from build123d import *

# Parameters (mm, degrees)
RESSALTO_EXTRUS_O1_DEPTH = 55
ESBO_O3_W                = 15
ESBO_O3_H                = 5
ESBO_O3_R                = 1.65
RESSALTO_EXTRUS_O2_DEPTH = 10


with BuildPart() as part:
    # Esboço1 → Ressalto-extrusão1 (new body)
    with BuildSketch(Plane.XY):
        with BuildLine():
            Line((0, 35), (0, -35))
            Line((0, -35), (13.5, -35))
            ThreePointArc((13.5, -35), (15.581665999, -34.780933834), (17.572127481, -34.133333333))
            Line((17.572127481, -34.133333333), (16.554095611, -31.85))
            ThreePointArc((16.554095611, -31.85), (6, -25), (16.554095611, -18.15))
            Line((16.554095611, -18.15), (17.572127481, -15.866666667))
            ThreePointArc((17.572127481, -15.866666667), (15.581665999, -15.219066166), (13.5, -15))
            Line((13.5, -15), (6, -15))
            Line((6, -15), (6, 15))
            Line((6, 15), (13.5, 15))
            ThreePointArc((13.5, 15), (15.581665999, 15.219066166), (17.572127481, 15.866666667))
            Line((17.572127481, 15.866666667), (16.554095611, 18.15))
            ThreePointArc((16.554095611, 18.15), (6, 25), (16.554095611, 31.85))
            Line((16.554095611, 31.85), (17.572127481, 34.133333333))
            ThreePointArc((17.572127481, 34.133333333), (15.581665999, 34.780933834), (13.5, 35))
            Line((13.5, 35), (0, 35))
        make_face()
    extrude(amount=RESSALTO_EXTRUS_O1_DEPTH)

    # Esboço3 → Ressalto-extrusão2 (add)
    with BuildSketch(Plane(origin=(6, 0, 0), x_dir=(0, 0, -1), z_dir=(1, 0, 0))):
        with Locations((-43.5, 15)):
            Rectangle(ESBO_O3_W, ESBO_O3_H)
        with Locations((-47.5, 15)):
            Circle(ESBO_O3_R, mode=Mode.SUBTRACT)
        with Locations((-39.5, 15)):
            Circle(ESBO_O3_R, mode=Mode.SUBTRACT)
    extrude(amount=RESSALTO_EXTRUS_O2_DEPTH)


solid = part.part
The model under review builds one solid part; all positions refer to its coordinate system, in mm. A direction names the side the tool comes from. Give positions to 0.01 mm unless a question says otherwise; leave off trailing zeros. Write each loop counter-clockwise with the first axis right and the second up, starting at its lowest first coordinate (ties: lowest second). Pieces come first, ordered by that corner, then holes.
1. Add section A-A, the plane x = 12.75. Write out the cut boundary in (y, z), plus the area to 3 significant figures.
2. Wall thickness on L1, parallel to Y at x = 13.5, z = 34; L2, parallel to Y at x = 8.25, z = 49.5; L3, parallel to Y at x = 9.25, z = 47.5: over which ranges is each line inside the solid? List them lowest first.
3. For P1, Ø10, axis at y = -4, z = 33.5, coming from the +X side; P2, Ø5, axis at x = 9, y = 1.5, coming from the +Z side; P3, Ø0.8, axis at x = 12, y = 13.5, coming from the +Z side; P4, Ø1.4, axis at x = 8.5, y = 13.5, coming from the -Z side, all flat-tipped, find the tip position at first contact; note any pin that passes through.
4. Tool access review of faces 4 (the flat face through (10, 15, 18)), 5 (the flat face through (17.06, 32.98, 27.12)), 6 (the cylindrical face through (15.553, 15.213, 27.115)): name each direction out of +Z, -Z, +X, -X, +Y, -Y from which nothing blocks a thin tool from reaching the whole face with its end or side.
5. Add section B-B, the plane z = 39.5. Write out the cut boundary in (x, y).
6. Add section C-C, the plane x = 7.75. Write out the cut boundary in (y, z), plus the area to 3 significant figures.
7. Add section D-D, the plane y = 25. Write out the cut boundary in (x, z).
8. Draft analysis for pull direction Z (two halves, no side actions). For faces 1 (the flat face through (6, 14, 39)), 2 (the flat face through (17.07, 16.99, 27.12)), 3 (the flat face through (11, 14, 36)), state which applies: +Z half, -Z half, draft (parallel to the pull), parting line (faces both ways), or undercut.
Worked answers:
1. outline: (-35, 0) - (-32.46, 0) - (-32.46, 55) - (-35, 55) - close; (-17.54, 0) - (-15, 0) - (-15, 55) - (-17.54, 55) - close; (12.5, 36) - (15, 36) - (15, 0) - (17.54, 0) - (17.54, 55) - (15, 55) - (15, 51) - (12.5, 51) - close; (32.46, 0) - (35, 0) - (35, 55) - (32.46, 55) - close; hole (15, 37.85) - (15, 41.15) arc R1.65 ccw to start; hole (15, 45.85) - (15, 49.15) arc R1.65 ccw to start
1. area: 587 mm2
2. L1: y = -35 to -32.5, -17.5 to -15, 15 to 17.5, 32.5 to 35
2. L2: y = -35 to -30.36, -19.64 to -15, 12.5 to 19.64, 30.36 to 35
2. L3: y = -35 to -31.18, -18.82 to -15, 12.5 to 13.35, 15 to 18.82, 31.18 to 35
3. P1: stops at x = 6
3. P2: passes through
3. P3: stops at z = 51
3. P4: stops at z = 36
4. face 4: -Z, +X
4. face 5: +Z, -Z, +X
4. face 6: +X
5. outline: (0, -35) - (13.5, -35) arc R10 ccw to (17.57, -34.13) - (16.55, -31.85) arc R7.5 cw (long way) to (16.55, -18.15) - (17.57, -15.87) arc R10 ccw to (13.5, -15) - (6, -15) - (6, 12.5) - (16, 12.5) - (16, 13.35) - (6, 13.35) - (6, 15) - (13.5, 15) arc R10 ccw to (17.57, 15.87) - (16.55, 18.15) arc R7.5 cw (long way) to (16.55, 31.85) - (17.57, 34.13) arc R10 ccw to (13.5, 35) - (0, 35) - close
6. outline: (-35, 0) - (-29.82, 0) - (-29.82, 55) - (-35, 55) - close; (-20.18, 0) - (-15, 0) - (-15, 55) - (-20.18, 55) - close; (12.5, 36) - (15, 36) - (15, 0) - (20.18, 0) - (20.18, 55) - (15, 55) - (15, 51) - (12.5, 51) - close; (29.82, 0) - (35, 0) - (35, 55) - (29.82, 55) - close; hole (15, 37.85) - (15, 41.15) arc R1.65 ccw to start; hole (15, 45.85) - (15, 49.15) arc R1.65 ccw to start
6. area: 1,170 mm2
7. outline: (0, 0) - (6, 0) - (6, 55) - (0, 55) - close
8. face 1: undercut
8. face 2: draft
8. face 3: -Z half
